Geometry check sheet. Reference: drawing and pictorial views, mm from the part's lowest x, y, z. Coordinates: 2 decimals unless noted, no trailing zeros. Write each loop counter-clockwise with the first axis right and the second up, starting at its lowest first coordinate (ties: lowest second). Pieces come first, ordered by that corner, then holes. Notation, with made-up numbers: (23.25, 87.5) -> (52.25, 87.5) arc R11 ccw to (52.25, 100.5) -> close; hole circle Ø3 at (71.5, 31). An arc over 180 degrees is marked (long way). Put each result on its own line as item: value.
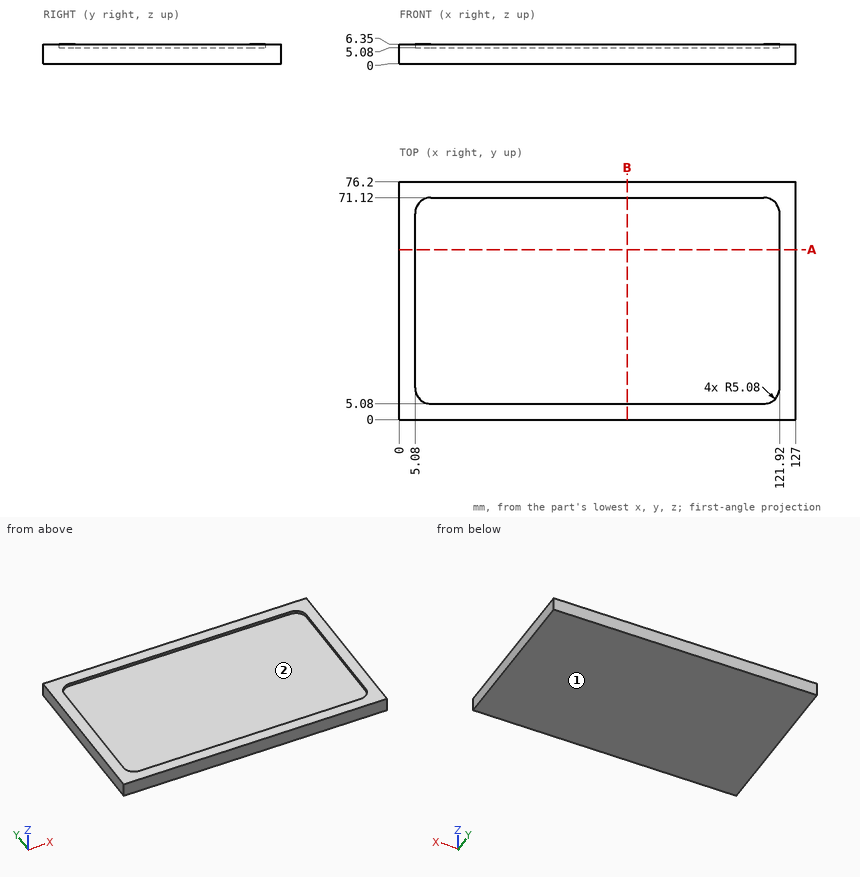
Q1. Mould release check, pull along X, two halves, no side actions. Record for the marked faces 1 and 2: released by +X, released by -X, zero draft, split by the parting line, or undercut.
Recorded:
face 1: zero draft
face 2: undercut
Q2. Depth check by flat-ended pin: P1, Ø20, axis at x = 78.5, y = 48, coming from the +Z side; P2, Ø0.6, axis at y = 51, z = 5.5, coming from the -X side. Enter the tip coordinate at first touch or a pass-through.
Recorded:
P1: stops at z = 5.08
P2: stops at x = 0
Q3. Cross-section at B-B (x = 73). Record the cut outline in (y, z).
Recorded:
outline: (0, 0) -> (76.2, 0) -> (76.2, 6.35) -> (71.12, 6.35) -> (71.12, 5.08) -> (5.08, 5.08) -> (5.08, 6.35) -> (0, 6.35) -> close
Q4. Cross-section at A-A (y = 54.5). Record the cut outline in (x, z), plus the area to 3 significant figures.
Recorded:
outline: (0, 0) -> (127, 0) -> (127, 6.35) -> (121.92, 6.35) -> (121.92, 5.08) -> (5.08, 5.08) -> (5.08, 6.35) -> (0, 6.35) -> close
area: 658 mm2
Q5. Material ranges on line 1 along X through (y, z) = (20, 5.25); line 2 along Z through (x, y) = (93.5, 65.5); line 3 along Y through (x, z) = (94, 5.75), recorded low to high.
Recorded:
line 1: x = 0 to 5.08, 121.92 to 127
line 2: z = 0 to 5.08
line 3: y = 0 to 5.08, 71.12 to 76.2
